Verification items for the finished model (mm, model axes). Face numbers are marked on the shaded views. A direction names the side the tool comes from. Round coordinates to 2 decimals unless told otherwise and drop trailing zeros. Write each loop counter-clockwise with the first axis right and the second up, starting at its lowest first coordinate (ties: lowest second). Pieces come first, ordered by that corner, then holes. Notation, with made-up numbers: (55.25, 87) -> (102.25, 87) arc R28 cw to (102.25, 110) -> close; hole circle Ø3 at (86, 11). An arc over 180 degrees is marked (long way). Answer as a JSON object with one key per item and string values. Group by question number.
(1) Set-up check for the marked faces 1, 2, 3 and 4: record each of +Z, -Z, +X, -X, +Y, -Y from which the full face is reachable in a straight line by a thin tool's end or side.
(2) Sectioned sample at C-C on x = -38.5. Count the separate pieces of the cut face and the enclosed holes in it, and give its area (3 significant figures).
(3) Sectioned sample at A-A on y = -1.5. Record the cut outline in (x, z), and give its area (3 significant figures).
(4) Draft check along X on the marked faces 5, 6 and 7. Enter one of: released by +X, released by -X, zero draft, split by the parting line, or undercut.
(5) Sectioned sample at B-B on z = 9.75. Record the cut outline in (x, y), and give its area (3 significant figures).
(6) Scan lines: L1, parallel to X at y = -6.35, z = 10.9; L2, parallel to Y at x = -39.5, z = 30.75; L3, parallel to Z at x = -19, y = -0.75. Record each from-to range of solid material in increasing order. Write a range as from..to.
(7) Gauge pin test, flat ends, axial feed: pin 1 Ø1.5 at (x, y) = (-60, -4.5) entering from +Z; pin 2 Ø4.5 at (x, y) = (-22.73, -6.35) entering from -Z; pin 3 Ø1.5 at (y, z) = (-6, 25) entering from -X. Record the tip position at first contact, or that the pin passes through.
```python
from build123d import *

# Parameters (mm, degrees)
F0_R      = 7.874
F1_DEPTH  = 12.7
F3_D      = 3.5687
F2_R      = 2.3876
F4_DEPTH  = 3.81
F6_R      = 3.175
F7_DEPTH  = 12.7
F9_D      = 3.9878
F9_DEPTH  = 6.35
F9_TIP    = 1.1980559883
F10_SIZE2 = 0.508
F10_SIZE  = 0.508


with BuildPart() as f1:
    # F0 (on Front) → F1 (new body)
    with BuildSketch(Plane.XZ):
        with BuildLine():
            Line((-60.8324925442, 14.3403462902), (-60.8324925442, 7.9903462902))
            Line((-60.8324925442, 7.9903462902), (-16.3824925442, 7.9903462902))
            Line((-16.3824925442, 7.9903462902), (-16.3824925442, 14.3403462902))
            Line((-16.3824925442, 14.3403462902), (-19.0494925442, 14.3403462902))
            ThreePointArc((-19.0494925442, 14.3403462902), (-23.5396206047, 16.2002182296), (-25.3994925442, 20.6903462902))
            Line((-25.3994925442, 20.6903462902), (-25.3994925442, 22.2143462902))
            ThreePointArc((-25.3994925442, 22.2143462902), (-28.2264978922, 29.0393409422), (-35.0514925442, 31.8663462902))
            Line((-35.0514925442, 31.8663462902), (-41.9094925442, 31.8663462902))
            ThreePointArc((-41.9094925442, 31.8663462902), (-48.7344871962, 29.0393409422), (-51.5614925442, 22.2143462902))
            Line((-51.5614925442, 22.2143462902), (-51.5614925442, 20.6903462902))
            ThreePointArc((-51.5614925442, 20.6903462902), (-53.4213644836, 16.2002182296), (-57.9114925442, 14.3403462902))
            Line((-57.9114925442, 14.3403462902), (-60.8324925442, 14.3403462902))
        make_face()
        with Locations((-38.4804925442, 20.6903462902)):
            Circle(F0_R, mode=Mode.SUBTRACT)
    extrude(amount=F1_DEPTH)

    # F3 (through all)
    with Locations(Plane(origin=(0, 0, 7.9903462902), x_dir=(1, 0, 0), z_dir=(0, 0, -1))):
        with Locations((-54.4824925442, 6.35), (-22.7324925442, 6.35)):
            Hole(F3_D / 2)

    # F2 (on face) → F4 (cut)
    with BuildSketch(Plane(origin=(0, 0, 7.9903462902), x_dir=(1, 0, 0), z_dir=(0, 0, -1))):
        with Locations((-54.4824925442, 6.35)):
            Circle(F2_R)
        with Locations((-22.7324925442, 6.35)):
            Circle(F2_R)
    extrude(amount=-F4_DEPTH, mode=Mode.SUBTRACT)

    # F6 (on offset) → F7 (cut)
    with BuildSketch(Plane.XY.offset(27.0403462902)):
        with Locations((-54.4824925442, -6.35)):
            Circle(F6_R)
        with Locations((-22.7324925442, -6.35)):
            Circle(F6_R)
    extrude(amount=-F7_DEPTH, mode=Mode.SUBTRACT)

    # F9
    with Locations(Plane.XY.offset(31.8663462902)):
        with Locations((-38.4804925442, -6.35)):
            Hole(F9_D / 2, depth=F9_DEPTH)
            with Locations((0, 0, -(F9_DEPTH + F9_TIP / 2))):  # 118° drill point
                Cone(0, F9_D / 2, F9_TIP, mode=Mode.SUBTRACT)

    # F10
    f10_edges = [f1.edges().sort_by_distance(p)[0] for p in [
        (-46.354493, 0, 20.690346),
    ]]
    chamfer(f10_edges, length=F10_SIZE, length2=F10_SIZE2)


solid = f1.part
```
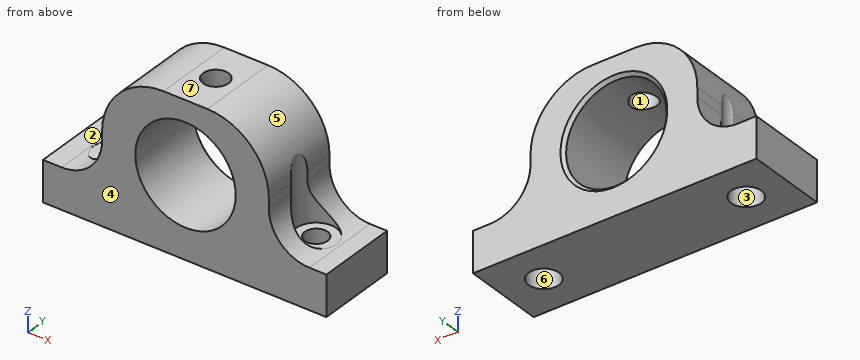
Computed values:
{
 "1": {"face 1": "+Z", "face 2": "+Z, -X, +Y, -Y", "face 3": "-Z", "face 4": "+Z, -Z, +X, -X, -Y"},
 "2": {"separate pieces": "3", "enclosed holes": "0", "area": "89.8 mm2"},
 "3": {"outline": "(-60.83, 7.99) -> (-16.38, 7.99) -> (-16.38, 14.34) -> (-19.05, 14.34) arc R6.35 cw to (-25.4, 20.69) -> (-25.4, 22.21) arc R9.65 ccw to (-35.05, 31.87) -> (-41.91, 31.87) arc R9.65 ccw to (-51.56, 22.21) -> (-51.56, 20.69) arc R6.35 cw to (-57.91, 14.34) -> (-60.83, 14.34) -> close; hole circle Ø15.75 at (-38.48, 20.69)", "area": "523 mm2"},
 "4": {"face 5": "released by +X", "face 6": "undercut", "face 7": "zero draft"},
 "5": {"outline": "(-60.83, -12.7) -> (-16.38, -12.7) -> (-16.38, 0) -> (-60.83, 0) -> close; hole circle Ø4.78 at (-54.48, -6.35); hole circle Ø4.78 at (-22.73, -6.35)", "area": "529 mm2"},
 "6": {"L1": "-60.83..-56.87, -52.09..-25.12, -20.34..-16.38", "L2": "-12.7..-8.06, -4.64..0", "L3": "7.99..14.34"},
 "7": {"pin 1": "z = 14.34", "pin 2": "z = 11.8", "pin 3": "x = -51.34"}
}
